```python
from build123d import *

# Parameters (mm, degrees)
SKETCH_1_R      = 2.15
SKETCH_1_R_2    = 1.75
EXTRUDE_1_DEPTH = 495


with BuildPart() as part:
    # 草图1 → 凸台-拉伸1 (new body)
    # profile 1 of 5: a face of its own
    with BuildSketch(Plane(origin=(0, 0, 0), x_dir=(1, 0, 0), z_dir=(0, 1, 0))):
        Polygon((-2.2, 8.7), (-2.2, 10), (-10, 10), (-10, 2.2), (-8.7, 2.2), (-8.7, 4.05), (-4.7, 4.05), (-4.7, 2.2), (-2.95, 2.2), (-2.95, 2.95), (-2.2, 2.95), (-2.2, 4.7), (-4.05, 4.7), (-4.05, 8.7), align=None)
        with Locations(Location((-6.9, 6.9, 0), (0, 0, 270))):
            Circle(SKETCH_1_R, mode=Mode.SUBTRACT)
    # profile 2 of 5: a face of its own
    with BuildSketch(Plane(origin=(0, 0, 0), x_dir=(1, 0, 0), z_dir=(0, 1, 0))):
        Polygon((2.2, 2.95), (-2.2, 2.95), (-2.95, 2.95), (-2.95, 2.2), (-2.95, -2.2), (-2.95, -2.95), (-2.2, -2.95), (2.2, -2.95), (2.95, -2.95), (2.95, -2.2), (2.95, 2.2), (2.95, 2.95), align=None)
        with Locations(Location((0, 0, 0), (0, 0, 270))):
            Circle(SKETCH_1_R_2, mode=Mode.SUBTRACT)
    # profile 3 of 5: a face of its own
    with BuildSketch(Plane(origin=(0, 0, 0), x_dir=(1, 0, 0), z_dir=(0, 1, 0))):
        Polygon((-8.7, -2.2), (-10, -2.2), (-10, -10), (-2.2, -10), (-2.2, -8.7), (-4.05, -8.7), (-4.05, -4.7), (-2.2, -4.7), (-2.2, -2.95), (-2.95, -2.95), (-2.95, -2.2), (-4.7, -2.2), (-4.7, -4.05), (-8.7, -4.05), align=None)
        with Locations(Location((-6.9, -6.9, 0), (0, 0, 270))):
            Circle(SKETCH_1_R, mode=Mode.SUBTRACT)
    # profile 4 of 5: a face of its own
    with BuildSketch(Plane(origin=(0, 0, 0), x_dir=(1, 0, 0), z_dir=(0, 1, 0))):
        Polygon((10, -10), (10, -2.2), (8.7, -2.2), (8.7, -4.05), (4.7, -4.05), (4.7, -2.2), (2.95, -2.2), (2.95, -2.95), (2.2, -2.95), (2.2, -4.7), (4.05, -4.7), (4.05, -8.7), (2.2, -8.7), (2.2, -10), align=None)
        with Locations(Location((6.9, -6.9, 0), (0, 0, 270))):
            Circle(SKETCH_1_R, mode=Mode.SUBTRACT)
    # profile 5 of 5: a face of its own
    with BuildSketch(Plane(origin=(0, 0, 0), x_dir=(1, 0, 0), z_dir=(0, 1, 0))):
        Polygon((10, 10), (2.2, 10), (2.2, 8.7), (4.05, 8.7), (4.05, 4.7), (2.2, 4.7), (2.2, 2.95), (2.95, 2.95), (2.95, 2.2), (4.7, 2.2), (4.7, 4.05), (8.7, 4.05), (8.7, 2.2), (10, 2.2), align=None)
        with Locations(Location((6.9, 6.9, 0), (0, 0, 270))):
            Circle(SKETCH_1_R, mode=Mode.SUBTRACT)
    extrude(amount=-EXTRUDE_1_DEPTH)


solid = part.part
```
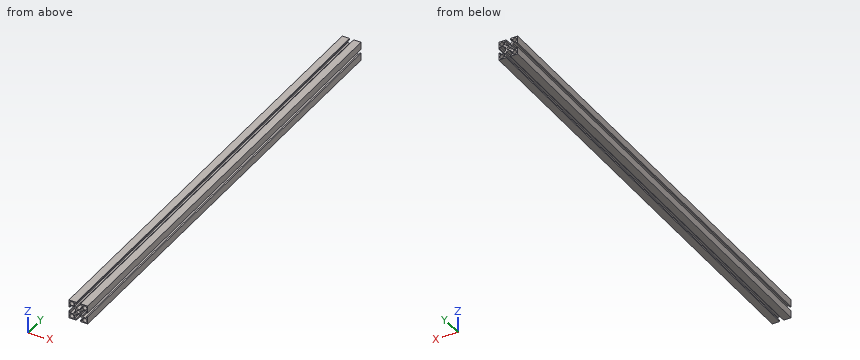
For this review, take the finished solid that the model builds, in its own axes (mm). Coordinates: 2 decimals unless noted, no trailing zeros. Answer in a Markdown table with one row per item. Add a question column.
Q1. We need section A-A, the plane y = -107. Count the separate pieces of the cut face and the enclosed holes in it, and give its area (3 significant figures).
Q2. For probe 1 along X at (y, z) = (-417, -7.25); probe 2 along Z at (x, y) = (-6.75, -123); probe 3 along Z at (x, y) = (3.25, -51.5), list the stretches that pass through material, from the lowest coordinate up.
Q3. For P1, Ø4, axis at x = 0, z = 0, coming from the -Y side; P2, Ø2, axis at y = -368, z = 0.5, coming from the +X side; P3, Ø2, axis at y = -360, z = 1, coming from the -X side, all flat-tipped, find the tip position at first contact; note any pin that passes through.
Answer list:
| question | item | result |
|---|---|---|
| 1 | separate pieces | 1 |
| 1 | enclosed holes | 5 |
| 1 | area | 149 mm2 |
| 2 | probe 1 | x = -10 to -9.02, -4.78 to -4.05, 4.05 to 4.78, 9.02 to 10 |
| 2 | probe 2 | z = -10 to -9.04, -4.76 to -4.05, 4.05 to 4.76, 9.04 to 10 |
| 2 | probe 3 | z = -10 to -8.7, -4.7 to -2.2, 2.2 to 4.7, 8.7 to 10 |
| 3 | P1 | stops at y = -495 |
| 3 | P2 | stops at x = 2.95 |
| 3 | P3 | stops at x = -2.95 |
